Check sheet for the modelled part. Datum: model origin and axes. Units: mm. Face numbers are marked on the shaded views. Give positions to 0.01 mm unless a question says otherwise; leave off trailing zeros. Order: outer loops, then holes, each group sorted by start corner. A loop starts at its lowest first (then second) coordinate and runs counter-clockwise, first axis right, second up.
Item 1: Gauge pin test, flat ends, axial feed: P1, Ø1.5, axis at x = -8.5, z = 3.5, coming from the -Y side; P2, Ø4, axis at x = -57, z = 2.5, coming from the -Y side; P3, Ø2, axis at x = 30.5, z = 1.5, coming from the -Y side. Record the tip position at first contact, or that the pin passes through.
Item 2: Sectioned sample at C-C on z = 4.5. Record the boundary of the cut face in (x, y), and give its area (3 significant figures).
Item 3: Material ranges on line 1 along Y through (x, z) = (0, 4.25); line 2 along X through (y, z) = (1, 1.75); line 3 along X through (y, z) = (9, 4.5), recorded low to high.
Item 4: Sectioned sample at D-D on y = 5. Record the boundary of the cut face in (x, z).
Item 5: Sectioned sample at B-B on y = -7. Record the boundary of the cut face in (x, z).
Item 6: Sectioned sample at A-A on x = -75. Record the boundary of the cut face in (y, z).
Item 7: Release check for a two-part mould opening along X. For the marked faces 1, 2 and 3 record: released by +X, released by -X, zero draft, split by the parting line, or undercut.
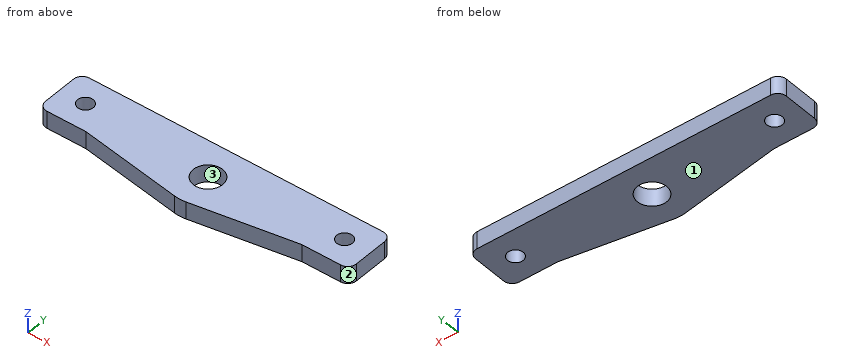
from build123d import *

# Parameters (mm, degrees)
F0_R     = 4.5
F0_R_2   = 8.5
F1_DEPTH = 10
F2_R     = 5


with BuildPart() as f1:
    # F0 (on Top) → F1 (new body)
    with BuildSketch(Plane.XY):
        with BuildLine():
            Line((-90, 20), (-90, -10))
            Line((-90, -10), (-62.5, -10))
            Line((-62.5, -10), (-17.3205080757, -10))
            ThreePointArc((-17.3205080757, -10), (-17.3205080604, 10.0000000264), (6.11e-08, 20))
            Line((6.11e-08, 20), (-90, 20))
        make_face()
        with Locations((-75, 5)):
            Circle(F0_R, mode=Mode.SUBTRACT)
        with BuildLine():
            Line((-17.3205080757, -10), (-62.5, -10))
            Line((-62.5, -10), (-3.2423308207, -19.7354323705))
            ThreePointArc((-3.2423308207, -19.7354323705), (-11.3755108338, -16.4498557219), (-17.3205080757, -10))
        make_face()
        with BuildLine():
            ThreePointArc((6.11e-08, 20), (-17.3205080604, 10.0000000264), (-17.3205080757, -10))
            Line((-17.3205080757, -10), (17.3205080757, -10))
            ThreePointArc((17.3205080757, -10), (19.3185165258, -5.1763809021), (20, 0))
            ThreePointArc((20, 0), (14.1421356453, 14.1421356021), (6.11e-08, 20))
        make_face()
        Circle(F0_R_2, mode=Mode.SUBTRACT)
        with BuildLine():
            Line((17.3205080757, -10), (-17.3205080757, -10))
            ThreePointArc((-17.3205080757, -10), (-11.3755108338, -16.4498557219), (-3.2423308207, -19.7354323705))
            ThreePointArc((-3.2423308207, -19.7354323705), (0, -20), (3.2423308207, -19.7354323705))
            ThreePointArc((3.2423308207, -19.7354323705), (11.3755108338, -16.4498557219), (17.3205080757, -10))
        make_face()
        with BuildLine():
            Line((90, 20), (6.11e-08, 20))
            ThreePointArc((6.11e-08, 20), (14.1421356453, 14.1421356021), (20, 0))
            ThreePointArc((20, 0), (19.3185165258, -5.1763809021), (17.3205080757, -10))
            Line((17.3205080757, -10), (62.5, -10))
            Line((62.5, -10), (90, -10))
            Line((90, -10), (90, 20))
        make_face()
        with Locations((75, 5)):
            Circle(F0_R, mode=Mode.SUBTRACT)
        with BuildLine():
            Line((62.5, -10), (17.3205080757, -10))
            ThreePointArc((17.3205080757, -10), (11.3755108338, -16.4498557219), (3.2423308207, -19.7354323705))
            Line((3.2423308207, -19.7354323705), (62.5, -10))
        make_face()
    extrude(amount=F1_DEPTH)

    # F2
    f2_edges = [f1.edges().sort_by_distance(p)[0] for p in [
        (-90, -10, 5),
        (90, -10, 5),
        (-90, 20, 5),
        (90, 20, 5),
    ]]
    fillet(f2_edges, radius=F2_R)


solid = f1.part
Report:
1. P1: stops at y = -18.99
1. P2: stops at y = -11.23
1. P3: stops at y = -15.42
2. outline: (-90, -5) arc R5 ccw to (-85, -10) - (-62.5, -10) - (-3.24, -19.74) arc R20 ccw to (3.24, -19.74) - (62.5, -10) - (85, -10) arc R5 ccw to (90, -5) - (90, 15) arc R5 ccw to (85, 20) - (-85, 20) arc R5 ccw to (-90, 15) - close; hole circle Ø9 at (-75, 5); hole circle Ø17 at (0, 0); hole circle Ø9 at (75, 5)
2. area: 5,670 mm2
3. line 1: y = -20 to -8.5, 8.5 to 20
3. line 2: x = -90 to -77.06, -72.94 to -8.44, 8.44 to 72.94, 77.06 to 90
3. line 3: x = -90 to -77.06, -72.94 to 72.94, 77.06 to 90
4. outline: (-90, 0) - (-79.5, 0) - (-79.5, 10) - (-90, 10) - close; (-70.5, 0) - (-6.87, 0) - (-6.87, 10) - (-70.5, 10) - close; (6.87, 0) - (70.5, 0) - (70.5, 10) - (6.87, 10) - close; (79.5, 0) - (90, 0) - (90, 10) - (79.5, 10) - close
5. outline: (-89.58, 0) - (-4.82, 0) - (-4.82, 10) - (-89.58, 10) - close; (4.82, 0) - (89.58, 0) - (89.58, 10) - (4.82, 10) - close
6. outline: (-10, 0) - (0.5, 0) - (0.5, 10) - (-10, 10) - close; (9.5, 0) - (20, 0) - (20, 10) - (9.5, 10) - close
7. face 1: zero draft
7. face 2: released by +X
7. face 3: undercut
